Geometry: final body of the model. Coordinates: model frame, mm. A direction names the side the tool comes from. Coordinates: 2 decimals unless noted, no trailing zeros. Loops run counter-clockwise (first coordinate to the right, second up) from the corner with the lowest first, then second, coordinate; pieces in that order, holes last. Notation, with made-up numbers: (-28, -10) - (10, -10) arc R27 cw to (10, 26) - close; hole circle Ø10 at (88, 33). An arc over 180 degrees is marked (long way). Return JSON: item names as keys, results as strings.
from build123d import *

# Parameters (mm, degrees)
F0_R          = 6.75
F0_R_2        = 33
F0_R_3        = 7
F0_R_4        = 27.48975
F1_DEPTH      = 19.5
F1_DEPTH_BACK = 19.5
F2_START      = 15
F2_DEPTH      = 10
F6_DEPTH      = 12.5
F6_DEPTH_BACK = 12.5
F7_R          = 3
F8_SIZE       = 0.5
F9_R          = 0.5


# Not quite as in the source:
# - a feature names something its author has since deleted; it is built from what else it names


with BuildPart() as f1:
    # F0 (on Top) → F1 (new body, two sides)
    with BuildSketch(Plane.XY) as f1_sk:
        with BuildLine():
            Line((-19.4499833155, -81.9024031138), (107.1556085776, -13.1832191017))
            ThreePointArc((107.1556085776, -13.1832191017), (114.9775485096, 0.8203905436), (105.6729061946, 13.8858969933))
            Line((105.6729061946, 13.8858969933), (-27.583481298, 68.3260953068))
            ThreePointArc((-27.583481298, 68.3260953068), (-40.0371705269, 66.8836794016), (-45.4810708907, 55.5903677578))
            Line((-45.4810708907, 55.5903677578), (-38.6325816401, -71.1782300471))
            ThreePointArc((-38.6325816401, -71.1782300471), (-31.9952103295, -81.8240816881), (-19.4499833155, -81.9024031138))
        make_face()
        with Locations((-25.6515107494, -70.4769465589)):
            Circle(F0_R, mode=Mode.SUBTRACT)
        Circle(F0_R_2, mode=Mode.SUBTRACT)
        with Locations((-32.5, 56.291651246)):
            Circle(F0_R_3, mode=Mode.SUBTRACT)
        with Locations((63, 0)):
            Circle(F0_R_3, mode=Mode.SUBTRACT)
        with Locations((81.5, 0)):
            Circle(F0_R_3, mode=Mode.SUBTRACT)
        with Locations((100, 0)):
            Circle(F0_R_3, mode=Mode.SUBTRACT)
        Circle(F0_R_2)
        Circle(F0_R_4, mode=Mode.SUBTRACT)
    extrude(amount=F1_DEPTH)
    extrude(f1_sk.sketch, amount=-F1_DEPTH_BACK)


with BuildPart() as f2:
    # F0 (on Top) → F2 (new body)
    with BuildSketch(Plane.XY.offset(F2_START)):
        Circle(F0_R_2)
        Circle(F0_R_4, mode=Mode.SUBTRACT)
    extrude(amount=F2_DEPTH)


with BuildPart() as f3_1:
    # F3: instance of F2
    add(f2.part.mirror(Plane.XY))


with BuildPart() as f1_1:
    add(f1.part)

    # F4: cut F2, F3_1
    add(f2.part, mode=Mode.SUBTRACT)
    add(f3_1.part, mode=Mode.SUBTRACT)

    # F5 (on Top) → F6 (cut, two sides)
    with BuildSketch(Plane.XY) as f6_sk:
        Polygon((-66.9979324298, -150.1462552281), (233.1545138204, 12.7709657028), (-82.7719960075, 141.8387137572), (-75.4085285246, 5.5376386383), (45, 75.0555349947), (45, -74.9084380282), (-73.3904532444, -31.8178370259), align=None)
    extrude(amount=-F6_DEPTH, mode=Mode.SUBTRACT)
    extrude(f6_sk.sketch, amount=F6_DEPTH_BACK, mode=Mode.SUBTRACT)

    # F7
    f7_edges = [f1_1.edges().sort_by_distance(p)[0] for p in [
        (45, -4.12355, -12.5),
        (-17.833672, 38.778497, -12.5),
        (-17.833672, 38.778497, 12.5),
        (45, -4.12355, 12.5),
        (-12.985509, -53.803439, 12.5),
        (-12.985509, -53.803439, -12.5),
    ]]
    fillet(f7_edges, radius=F7_R)

    # F8
    f8_edges = [f1_1.edges().sort_by_distance(p)[0] for p in [
        (-27.48975, 0, 15),
        (-27.48975, 0, -15),
        (-33, 0, 19.5),
        (-33, 0, -19.5),
    ]]
    chamfer(f8_edges, length=F8_SIZE)

    # F9
    f9_edges = [f1_1.edges().sort_by_distance(p)[0] for p in [
        (-33, 0, -15),
        (-33, 0, 15),
    ]]
    fillet(f9_edges, radius=F9_R)


solid = f1_1.part
Item 1: Section query C-C, the plane x = 100. Return loops of the section in (y, z), and give its area (3 significant figures).
Worked out:
{"outline": "(-17.07, -19.5) - (-7, -19.5) - (-7, -12.5) - (-17.07, -12.5) - close; (-17.07, 12.5) - (-7, 12.5) - (-7, 19.5) - (-17.07, 19.5) - close; (7, -19.5) - (16.2, -19.5) - (16.2, -12.5) - (7, -12.5) - close; (7, 12.5) - (16.2, 12.5) - (16.2, 19.5) - (7, 19.5) - close", "area": "270 mm^2"}
Item 2: Mould query, pull axis Z, two halves, no side actions, for faces 1 (the face through (9, 27, -15)), 2 (the face through (-26.53, -63.784, -16.049)), 3 (the face through (-18.197, 38.569, 0.133)). Classes: +Z half, -Z half, draft (parallel to the pull), parting line (faces both ways), or undercut.
Worked out:
{"face 1": "-Z half", "face 2": "draft", "face 3": "undercut"}
Item 3: Reachability of faces 4 (the face through (45, -4, 0)), 5 (the face through (-21, -65, -12.5)), 6 (the face through (-26, 49, 12.5)) from +Z, -Z, +X, -X, +Y, -Y: full face, straight path, thin tool, end or side. Return the list, or none.
Worked out:
{"face 4": "+X, +Y, -Y", "face 5": "-X, -Y", "face 6": "-X, +Y"}
Item 4: Ray query, probe 1 along Z at (x, y) = (-3, -64); probe 2 along Y at (x, z) = (-10, 18); probe 3 along Y at (x, z) = (100, -16). Return the intervals inside material, ascending. Write a range as from..to.
Worked out:
{"probe 1": "-19.5..-12.5, 12.5..19.5", "probe 2": "-76.77..-31.45, 31.45..61.14", "probe 3": "-17.07..-7, 7..16.2"}
Item 5: Section query D-D, the plane y = 0. Count the separate pieces of the cut face and the enclosed holes in it, and give its area (3 significant figures).
Worked out:
{"separate pieces": "8", "enclosed holes": "0", "area": "1,560 mm^2"}
Item 6: Section query B-B, the plane x = 63. Return loops of the section in (y, z).
Worked out:
{"outline": "(-37.15, -19.5) - (-7, -19.5) - (-7, -12.5) - (-37.15, -12.5) - close; (-37.15, 12.5) - (-7, 12.5) - (-7, 19.5) - (-37.15, 19.5) - close; (7, -19.5) - (31.32, -19.5) - (31.32, -12.5) - (7, -12.5) - close; (7, 12.5) - (31.32, 12.5) - (31.32, 19.5) - (7, 19.5) - close"}
Item 7: First-contact query: pin 1 Ø22.5 at (x, y) = (63, 0) entering from -Z; pin 2 Ø5 at (x, z) = (-0.5, -5) entering from -Y; pin 3 Ø9.5 at (y, z) = (-22.5, 3) entering from +X; pin 4 Ø4 at (y, z) = (46.5, -10) entering from -X. Flat tips, straight axial feed; report the tip coordinate or a pass-through.
Worked out:
{"pin 1": "z = -19.5", "pin 2": "y = -59.26", "pin 3": "x = 45", "pin 4": "x = -8.29"}
Item 8: Section query A-A, the plane z = 5.5. Return loops of the section in (x, y), and give its area (3 significant figures).
Worked out:
{"outline": "(-43.76, 23.81) - (-40.1, -43.93) - (14.13, -63.67) - (45, -46.92) - (45, 38.67) - (8.1, 53.75) - close; hole circle Ø54.98 at (0, 0)", "area": "6,000 mm^2"}
